```python
from build123d import *

# Parameters (mm, degrees)
SKETCH_R        = 11
SKETCH_R_2      = 1.7
PAD_DEPTH       = 7
PAD001_DEPTH    = 6.9
SKETCH006_R     = 3.5
POCKET003_DEPTH = 10
SKETCH007_R     = 2.2
POCKET_DEPTH    = 6
SKETCH003_R     = 1.5
POCKET004_DEPTH = 7.3
CHAMFER_SIZE    = 1.7
CHAMFER001_SIZE = 1.7


with BuildPart() as part:
    # Sketch → Pad (new body)
    with BuildSketch(Plane.XY):
        Circle(SKETCH_R)
        with Locations((0, 6)):
            Circle(SKETCH_R_2, mode=Mode.SUBTRACT)
        with Locations((0, -6)):
            Circle(SKETCH_R_2, mode=Mode.SUBTRACT)
    extrude(amount=PAD_DEPTH)

    # Sketch004 → Pad001 (new body)
    with BuildSketch(Plane.XY.offset(7)):
        with BuildLine():
            Line((-3.35, 3.35), (3.35, 3.35))
            ThreePointArc((3.35, -3.35), (4.737615, 0), (3.35, 3.35))
            Line((3.35, -3.35), (-3.35, -3.35))
            ThreePointArc((-3.35, 3.35), (-4.737615, 0), (-3.35, -3.35))
        make_face()
    extrude(amount=PAD001_DEPTH)

    # Sketch006 → Pocket003 (cut)
    with BuildSketch(Plane.XY.offset(13.9)):
        with Locations((0, 6)):
            Circle(SKETCH006_R)
        with Locations((0, -6)):
            Circle(SKETCH006_R)
    extrude(amount=-POCKET003_DEPTH, mode=Mode.SUBTRACT)

    # Sketch007 → Pocket (cut)
    with BuildSketch(Plane(origin=(0, 0, 0), x_dir=(1, 0, 0), z_dir=(0, 0, -1))):
        Circle(SKETCH007_R)
    extrude(amount=-POCKET_DEPTH, mode=Mode.SUBTRACT)

    # Sketch003 → Pocket004 (cut)
    with BuildSketch(Plane.XY.offset(13.9)):
        Circle(SKETCH003_R)
    extrude(amount=-POCKET004_DEPTH, mode=Mode.SUBTRACT)

    # Chamfer
    chamfer_edges = [part.edges().sort_by_distance(p)[0] for p in [
        (-1.7, 6, 3.9),
    ]]
    chamfer(chamfer_edges, length=CHAMFER_SIZE)

    # Chamfer001
    chamfer001_edges = [part.edges().sort_by_distance(p)[0] for p in [
        (-1.7, -6, 3.9),
    ]]
    chamfer(chamfer001_edges, length=CHAMFER001_SIZE)


solid = part.part
```
Input: part model. Units: mm. Frame: model coordinates. A direction names the side the tool comes from. Coordinates: 2 decimals unless noted, no trailing zeros. Order: outer loops, then holes, each group sorted by start corner. A loop starts at its lowest first (then second) coordinate and runs counter-clockwise, first axis right, second up. Notation, with made-up numbers: (67.5, -6) - (103.5, -6) arc R31 ccw to (103.5, 18) - close; hole circle Ø7 at (59, 10.25). An arc over 180 degrees is marked (long way). Put each result on its own line as item: value.
1. Reachability of faces 4 (the face through (2.1, -0.66, 2.96)), 5 (the face through (-3, 3.35, 10)), 6 (the face through (-4.737, 0.052, 10.402)), 7 (the face through (0, 0, 6.6)), 8 (the face through (3, -3.35, 10)) from +Z, -Z, +X, -X, +Y, -Y: full face, straight path, thin tool, end or side. Return the list, or none.
Report:
face 4: -Z
face 5: +Z, +X, -X, +Y
face 6: +Z, -X
face 7: +Z
face 8: +Z, +X, -X, -Y
2. Line query: line 1 along Y through (x, z) = (1.5, 5.75); line 2 along Y through (x, z) = (0, 10.25); line 3 along Y through (x, z) = (-0.25, 4.25). Output: solid intervals per line, ascending.
Report:
line 1: y = -10.9 to -9.16, -2.84 to -1.61, 1.61 to 2.84, 9.16 to 10.9
line 2: y = -2.5 to -1.5, 1.5 to 2.5
line 3: y = -11 to -9.49, -2.51 to -2.19, 2.19 to 2.51, 9.49 to 11
3. Contact query for flat-ended pins moving along their axis: pin 1 Ø1.8 at (x, y) = (0, 0) entering from +Z; pin 2 Ø5.5 at (x, y) = (0, 6) entering from +Z; pin 3 Ø1 at (y, z) = (2.5, 3.5) entering from -X; pin 4 Ø2.5 at (x, y) = (0, 6) entering from +Z. Output: stop coordinate, or through.
Report:
pin 1: stops at z = 6.6
pin 2: stops at z = 3.25
pin 3: stops at x = -10.82
pin 4: passes through
4. Cut plane B-B on z = 11.5. Return the cut outline in (x, y), then the cut area to 3 significant figures.
Report:
outline: (-3.35, -3.35) - (-2.29, -3.35) arc R3.5 cw to (2.29, -3.35) - (3.35, -3.35) arc R4.74 ccw to (3.35, 3.35) - (2.29, 3.35) arc R3.5 cw to (-2.29, 3.35) - (-3.35, 3.35) arc R4.74 ccw to start; hole circle Ø3 at (0, 0)
area: 45.3 mm2
5. Draft query along X for faces 1 (the face through (-2.38, -10.74, 3.45)), 2 (the face through (0.971, 4.477, 2.306)), 3 (the face through (3, 3.35, 10)). Return one class per face: pulls with the +X half, pulls with the -X half, needs draft (parallel to the pull), parting line crosses it, or undercut.
Report:
face 1: parting line crosses it
face 2: undercut
face 3: needs draft
6. Cut plane D-D on z = 1.25. Return the cut outline in (x, y), then the cut area to 3 significant figures.
Report:
outline: circle Ø22 at (0, 0); hole circle Ø4.4 at (0, 0); hole circle Ø3.4 at (0, -6); hole circle Ø3.4 at (0, 6)
area: 347 mm2
7. Cut plane A-A on x = 0. State how many separate pieces and enclosed holes the cut face has, then the cut area to 3 significant figures.
Report:
separate pieces: 3
enclosed holes: 0
area: 64.5 mm2
8. Cut plane C-C on y = -6. Return the cut outline in (x, z), then the cut area to 3 significant figures.
Report:
outline: (-9.22, 0) - (-1.7, 0) - (-1.7, 2.2) - (-3.4, 3.9) - (-3.5, 3.9) - (-3.5, 7) - (-9.22, 7) - close; (1.7, 0) - (9.22, 0) - (9.22, 7) - (3.5, 7) - (3.5, 3.9) - (3.4, 3.9) - (1.7, 2.2) - close
area: 91.2 mm2
